The model under review builds one solid part; all positions refer to its coordinate system, in mm. A direction names the side the tool comes from. Round coordinates to 2 decimals unless told otherwise and drop trailing zeros. Order: outer loops, then holes, each group sorted by start corner. A loop starts at its lowest first (then second) coordinate and runs counter-clockwise, first axis right, second up. Notation, with made-up numbers: M 27.5,19.5 L 86.5,19.5 A20 cw 86.5,49.5 Z; hole C 56.5,-36 d1. An arc over 180 degrees is marked long. Use a Markdown table: item, result. Add a question column.
1. Insertion check: P1, Ø21, axis at x = -16, z = 0, coming from the +Y side; P2, Ø8, axis at y = 1, z = -2.5, coming from the -X side; P3, Ø3.5, axis at x = -23, z = 0, coming from the +Y side. Each pin has a flat end and moves straight along its axis. Give the tip position at first contact, or say it passes through.
2. The part is to be moulded in two halves that separate along Y. For faces 4 (the flat face through (2, -1, -17.75)), 5 (the flat face through (-19, -15, 0)), 6 (the cylindrical face through (-33.727, -12.972, 5.358)), 7 (the cylindrical face through (2.03, -6.25, 15.06)), say which applies: +Y half, -Y half, draft (parallel to the pull), parting line (faces both ways), or undercut.
3. Consider section A-A on x = -23. State the section outline as (y, z) points.
4. For faces 1 (the cylindrical face through (2.03, 4.75, -15.06)), 2 (the flat face through (0, 2, 0)), 3 (the flat face through (-14, -11.2, -22.5)), list the 3-axis set-ups (+Z, -Z, +X, -X, +Y, -Y) from which the entire face can be reached by the end or side of a thin tool; tool diameter is ignored.
5. To check wall thickness, follow probe 1 along Z at (x, y) = (-31, -12.1); probe 2 along X at (y, z) = (-12.2, -5); probe 3 along X at (y, z) = (-8.75, 8). State the ranges of each line that lie inside material, in increasing order.
6. Consider section D-D on y = 11. State the section outline as (x, z) points.
7. Consider section B-B on z = 0. State the section outline as (x, y) points, then the cut area to 3 significant figures.
8. Consider section C-C on z = 15. State the section outline as (x, y) points, then the cut area to 3 significant figures.
Autodesk Inventor part; units mm, degrees
ref_plane "YZ Plane" through (0, 0, 0) normal (1, 0, 0) x (0, 1, 0)
ref_plane "XZ Plane" through (0, 0, 0) normal (0, 1, 0) x (-1, 0, 0)
ref_plane "XY Plane" through (0, 0, 0) normal (0, 0, 1) x (1, 0, 0)
sketch "Skizze1" plane through (0, 0, 0) normal (1, 0, 0) x (0, 1, 0)
  line L0 (15, 22.5) -> (-15, 22.5)
  line L1 (-15, 22.5) -> (-15, -22.5)
  line L2 (-15, -22.5) -> (15, -22.5)
  line L3 (15, -22.5) -> (15, 22.5)
  line L4 (15, 22.5) -> (-15, -22.5) construction
  line L5 (-15, 22.5) -> (15, -22.5) construction
  point P0 (0, 0)
  dimension "d0" = 30
  dimension "d1" = 45
extrude "Extrusion1" add sketch "Skizze1" along normal blind 4
sketch "Skizze2" plane through (0, 0, 0) normal (-1, 0, 0) x (0, 0, 1)
  line L0 (-22.5, -15) -> (-22.5, 15)
  line L1 (-22.5, -11) -> (22.5, -11)
  line L2 (22.5, -11) -> (22.5, -15)
  line L3 (22.5, -15) -> (-22.5, -15)
  line L4 (-22.5, -15) -> (-22.5, -11)
  line L5 (22.5, -15) -> (-22.5, -15)
  point P0 (0, 0)
  dimension "d4" = 4
  dimension "d5" = 0
extrude "Extrusion2" add sketch "Skizze2" along normal blind 42
sketch "Skizze3" plane through (4, -15, -22.5) normal (0, -1, 0) x (1, 0, 0)
  line L0 (0, 22.5) -> (-45.8958, 22.5)
  line L1 (0, 45) -> (0, 0)
  line L2 (-46, 0) -> (-46, 45)
  point P0 (-4, 22.5)
  point P1 (-27, 22.5)
  point P2 (-35, 17.5)
  point P3 (-35, 27.5)
  point P4 (-46, 22.5)
  dimension "d15" = 27
  dimension "d17" = 10
  dimension "d18" = 35
  dimension "d19" = 0
  dimension "d21" = 5
hole "Bohrung1" at (-23, -15, 0) at (-31, -15, -5) at (-31, -15, 5) direction (0, 1, 0) diameter 5.5 depth 11.8 tip angle 118
sketch "Skizze5" plane through (0, 0, 0) normal (-1, 0, 0) x (0, 0, 1)
  line L0 (-22.5, -15) -> (22.5, -15)
  point P0 (0, 0)
  point P1 (15, -3.5)
  point P2 (-15, -3.5)
  point P3 (15, 2)
  point P4 (-15, 2)
  dimension "d29" = 30
  dimension "d30" = 15
  dimension "d31" = 11.5
  dimension "d32" = 11.5
  dimension "d33" = 15
  dimension "d34" = 30
  dimension "d35" = 5.5
  dimension "d36" = 5.5
hole "Bohrung2" at (0, -3.5, 15) at (0, -3.5, -15) at (0, 2, 15) at (0, 2, -15) direction (1, 0, 0) diameter 5.5 depth 11.8 tip angle 118
sketch "Skizze6" plane through (0, 0, 0) normal (-1, 0, 0) x (0, 0, 1)
  circle A0 centre (15, -3.5) radius 2.75
  line L0 (17.75, -3.5) -> (17.75, 2.2896)
  line L1 (12.25, -3.5) -> (12.25, 2.2896)
  circle A1 centre (-15, -3.5) radius 2.75
  line L2 (-12.25, -3.5) -> (-12.25, 2.2896)
  line L3 (-17.75, -3.5) -> (-17.75, 2)
  circle A2 centre (-15, 2) radius 2.75
  line L4 (17.75, -3.5) -> (12.25, -3.5)
  line L5 (17.75, 2.2896) -> (12.25, 2.2896)
  line L6 (-12.25, -3.5) -> (-17.75, -3.5)
  line L7 (-12.25, 2.2896) -> (-17.7347, 2.2896)
  circle A3 centre (-15, 2) radius 2.75
  point P0 (0, 0)
  point P1 (15, -0.75)
  point P2 (-15, -0.75)
  point P3 (-12.25, 2)
extrude "Extrusion3" cut sketch "Skizze6" against normal blind 6 contours A0 L1 L5 L0 | L3 A2 A1 | A1 A2 L2
properties part number "Montagewinkel für Spannelement"
Answer block:
| question | item | result |
|---|---|---|
| 1 | P1 | y = -11 |
| 1 | P2 | x = 0 |
| 1 | P3 | through |
| 2 | face 4 | undercut |
| 2 | face 5 | -Y half |
| 2 | face 6 | draft |
| 2 | face 7 | undercut |
| 3 | outline | M -15,-22.5 L -11,-22.5 L -11,-2.75 L -15,-2.75 Z; M -15,2.75 L -11,2.75 L -11,22.5 L -15,22.5 Z |
| 4 | face 1 | +X, -X |
| 4 | face 2 | +Z, -Z, -X, +Y |
| 4 | face 3 | -Z, +X, -X, +Y, -Y |
| 5 | probe 1 | -22.5 to -7.75, -2.25 to 2.25, 7.75 to 22.5 |
| 5 | probe 2 | -42 to -33.75, -28.25 to 4 |
| 5 | probe 3 | 0 to 4 |
| 6 | outline | M 0,-22.5 L 4,-22.5 L 4,22.5 L 0,22.5 Z |
| 7 | outline | M -42,-15 L -25.75,-15 L -25.75,-11 L -42,-11 Z; M -20.25,-15 L 4,-15 L 4,15 L 0,15 L 0,-11 L -20.25,-11 Z |
| 7 | area | 266 mm^2 |
| 8 | outline | M -42,-15 L 4,-15 L 4,-6.25 L 0,-6.25 L 0,-11 L -42,-11 Z; M 0,4.75 L 4,4.75 L 4,15 L 0,15 Z |
| 8 | area | 244 mm^2 |
